Autodesk Inventor part; units mm, degrees
ref_plane "YZ Plane" through (0, 0, 0) normal (1, 0, 0) x (0, 1, 0)
ref_plane "XZ Plane" through (0, 0, 0) normal (0, 1, 0) x (-1, 0, 0)
ref_plane "XY Plane" through (0, 0, 0) normal (0, 0, 1) x (1, 0, 0)
sketch "스케치1" plane through (0, 0, 0) normal (1, 0, 0) x (0, 1, 0)
  line L0 (0, 0) -> (72.5, 0)
  line L1 (72.5, 0) -> (72.5, -76.5)
  line L2 (72.5, -76.5) -> (0, -76.5)
  line L3 (0, -76.5) -> (0, 0)
  line L4 (2, -24) -> (71, -24)
  line L5 (71, -24) -> (71, 0)
  line L6 (71, 0) -> (2, 0)
  line L7 (2, 0) -> (2, -24)
  line L8 (13, -75) -> (71, -75)
  line L9 (71, -75) -> (71, -27)
  line L10 (71, -27) -> (13, -27)
  line L11 (13, -27) -> (13, -75)
  line L12 (71, -27) -> (71, -24)
  line L13 (71, -75) -> (71, -76.5)
  point P0 (71, 0)
  point P1 (2, 0)
  dimension "d1" = 69
  dimension "d3" = 58
  dimension "d4" = 1.5
  dimension "d5" = 3
  dimension "d6" = 24
  dimension "d7" = 48
  dimension "d8" = 1.5
  dimension "d9" = 2
extrude "돌출1" add sketch "스케치1" along normal blind 118 contours L0 L7 L4 L12 L10 L11 L8 L13 L2 L3 | L0 L5 L4 L7 | L8 L11 L10 L9
extrude "돌출2" cut sketch "스케치1" along normal blind 70 contours L8 L11 L10 L9
extrude "돌출3" cut sketch "스케치1" along normal blind 115 contours L0 L5 L4 L7
sketch "스케치2" plane through (0, 71, -76.5) normal (0, 1, 0) x (1, 0, 0)
  line L0 (118, 0) -> (118, -76.5)
  line L1 (0, 0) -> (118, 0)
  line L2 (70, -1.5) -> (70, -49.5)
  line L3 (70, -49.5) -> (0, -49.5)
  line L4 (74, 0) -> (118, 0)
  line L5 (118, 0) -> (118, -49.5)
  line L6 (118, -49.5) -> (74, -49.5)
  line L7 (74, -49.5) -> (74, 0)
  point P0 (0, -76.5)
  dimension "d16" = 4
extrude "돌출4" cut sketch "스케치2" against normal blind 113
sketch "스케치3" plane through (0, 0, 0) normal (-1, 0, 0) x (0, 0, 1)
  line L0 (0, 2) -> (-24, 2)
  line L1 (-24, 2) -> (-24, 71)
  line L2 (-27, 71) -> (-27, 13)
  line L3 (-27, 13) -> (-75, 13)
  line L4 (-75, 13) -> (-75, 71)
  line L5 (-24, 71) -> (0, 71)
  line L6 (0, 2) -> (0, 71)
  line L7 (0, 71) -> (-24, 71)
  line L8 (-24, 71) -> (-75, 71)
extrude "돌출5" add sketch "스케치3" against normal blind 3
sketch "스케치4" plane through (0, 0, 0) normal (0, 0, 1) x (1, 0, 0)
  line L0 (0, 71) -> (0, 0)
  line L1 (0, 0) -> (118, 0)
  line L2 (118, 71) -> (118, 0)
  line L3 (118, 71) -> (0, 71)
  line L4 (0, 0) -> (74, 0)
  line L5 (59, 0) -> (59, 71) construction
  line L6 (118, 35.5) -> (0, 35.5) construction
  line L7 (118, 40.5) -> (128, 40.5)
  line L8 (128, 40.5) -> (128, 30.5)
  line L9 (128, 30.5) -> (118, 30.5)
  line L10 (118, 30.5) -> (118, 40.5)
  circle A0 centre (123, 35.5) radius 2
  line L11 (54, 0) -> (64, 0)
  line L12 (64, 0) -> (64, -10)
  line L13 (64, -10) -> (54, -10)
  line L14 (54, -10) -> (54, 0)
  circle A1 centre (59, -5) radius 2
  line L15 (-10, 40.5) -> (0, 40.5)
  line L16 (0, 40.5) -> (0, 30.5)
  line L17 (0, 30.5) -> (-10, 30.5)
  line L18 (-10, 30.5) -> (-10, 40.5)
  circle A2 centre (-5, 35.5) radius 2
  point P0 (54, 0)
  dimension "d21" = 10
  dimension "d22" = 10
  dimension "d23" = 4
  dimension "d24" = 5
  dimension "d25" = 5
  dimension "d26" = 10
  dimension "d27" = 10
  dimension "d28" = 4
  dimension "d29" = 5
  dimension "d30" = 5
  dimension "d31" = 10
  dimension "d32" = 10
  dimension "d33" = 4
  dimension "d34" = 5
  dimension "d35" = 5
  dimension "d38" = 40.5
  dimension "d39" = 128
extrude "돌출6" add sketch "스케치4" against normal blind 3 contours L0 L17 L18 L15 | L7 L8 L9 L2 | L1 L12 L13 L14
properties part number "battery_base"
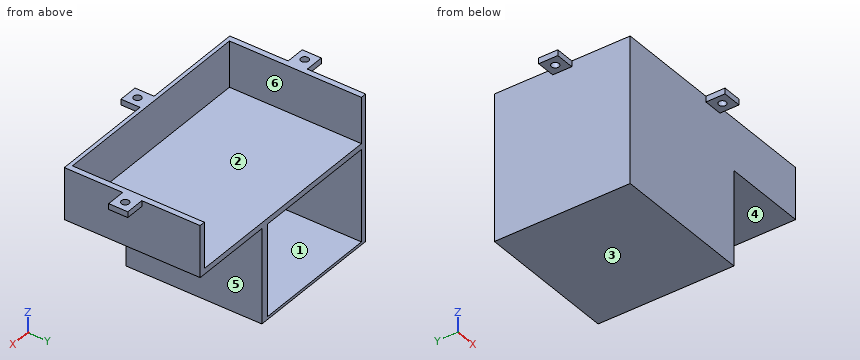
The model under review builds one solid part; all positions refer to its coordinate system, in mm. Face numbers are marked on the shaded views. A direction names the side the tool comes from. Round coordinates to 2 decimals unless told otherwise and drop trailing zeros. Write each loop counter-clockwise with the first axis right and the second up, starting at its lowest first coordinate (ties: lowest second). Pieces come first, ordered by that corner, then holes. Notation, with made-up numbers: M 8,71 L 34,71 A20 ccw 34,107 Z; hole C 56,88 d11. An arc over 180 degrees is marked long. Use CSV: the item, a comma, the result in double quotes. Start each with the question number.
(1) We need section C-C, the plane y = -5. State the section outline as (x, z) points.
(2) The part is to be moulded in two halves that separate along X. For the marked faces 4, 5 and 6, say which applies: +X half, -X half, draft (parallel to the pull), parting line (faces both ways), or undercut.
(3) We need section B-B, the plane x = 59. State the section outline as (y, z) points, then the cut area to 3 significant figures.
(4) For line 1 along X through (y, z) = (34, -35); line 2 along Z through (x, y) = (9, 62); line 3 along Y through (x, z) = (59, -1), list the stretches that pass through material, from the lowest coordinate up.
(5) We need section D-D, the plane z = -19. State the section outline as (x, y) points.
(6) Clearance check with flat-ended pins moving along their axes: P1, Ø11, axis at x = -7, y = 37.5, coming from the -Z side; P2, Ø0.9, axis at x = 121.5, z = -2, coming from the +Y side; P3, Ø10, axis at x = 23, z = -59.5, coming from the +Y side. State where each tip first meets the part, or that it passes through.
(7) Tool access review of the marked faces 1, 2 and 3: name each direction out of +Z, -Z, +X, -X, +Y, -Y from which nothing blocks a thin tool from reaching the whole face with its end or side.
(8) We need section A-A, the plane y = 35.5. State the section outline as (x, z) points, then the cut area to 3 significant figures.
Findings:
1,outline,"M 54,-3 L 57,-3 L 57,0 L 54,0 Z; M 61,-3 L 64,-3 L 64,0 L 61,0 Z"
2,face 4,"draft"
2,face 5,"+X half"
2,face 6,"undercut"
3,outline,"M -10,-3 L -7,-3 L -7,0 L -10,0 Z; M -3,-3 L 0,-3 L 0,-76.5 L 71,-76.5 L 71,-75 L 13,-75 L 13,-27 L 71,-27 L 71,-24 L 2,-24 L 2,0 L -3,0 Z"
3,area,"1,010 mm^2"
4,line 1,"0 to 3, 70 to 74"
4,line 2,"-76.5 to -75, -27 to -24"
4,line 3,"-10 to -7, -3 to 2"
5,outline,"M 0,0 L 118,0 L 118,71 L 115,71 L 115,2 L 3,2 L 3,71 L 0,71 Z"
6,P1,"z = -3"
6,P2,"y = 40.5"
6,P3,"y = 13"
7,face 1,"+Y"
7,face 2,"+Z, +Y"
7,face 3,"-Z, +X, -X, +Y, -Y"
8,outline,"M -10,-3 L -7,-3 L -7,0 L -10,0 Z; M -3,-3 L 0,-3 L 0,-76.5 L 74,-76.5 L 74,-27 L 118,-27 L 118,-3 L 121,-3 L 121,0 L 115,0 L 115,-24 L 3,-24 L 3,0 L -3,0 Z; M 125,-3 L 128,-3 L 128,0 L 125,0 Z; hole M 3,-75 L 70,-75 L 70,-27 L 3,-27 Z"
8,area,"981 mm^2"
